The listing builds one solid part. Answer for the finished solid, in the listing's coordinates (mm). A direction names the side the tool comes from. Round coordinates to 2 decimals unless told otherwise and drop trailing zeros. Write each loop counter-clockwise with the first axis right and the second up, starting at its lowest first coordinate (ties: lowest second). Pieces come first, ordered by that corner, then holes. Notation, with made-up numbers: (3.5, 1.5) - (54.5, 1.5) arc R30 ccw to (54.5, 39.5) - close; hole circle Ø9 at (84, 18). An arc over 180 degrees is marked (long way). Return JSON: item names as keys, results as strings. Group by question number.
from build123d import *

# Parameters (mm, degrees)
SKETCH_1_W      = 148
SKETCH_1_H      = 22
SKETCH_1_W_2    = 10
SKETCH_1_H_2    = 3
EXTRUDE_1_DEPTH = 3


with BuildPart() as part:
    # 草图1 → 凸台-拉伸1 (new body)
    with BuildSketch(Plane.XY):
        Rectangle(SKETCH_1_W, SKETCH_1_H)
        with Locations((-52, 7.5)):
            Rectangle(SKETCH_1_W_2, SKETCH_1_H_2, mode=Mode.SUBTRACT)
        with Locations((-67, 7.5)):
            Rectangle(SKETCH_1_W_2, SKETCH_1_H_2, mode=Mode.SUBTRACT)
        with Locations((-37, 7.5)):
            Rectangle(SKETCH_1_W_2, SKETCH_1_H_2, mode=Mode.SUBTRACT)
        with Locations((-22, 7.5)):
            Rectangle(SKETCH_1_W_2, SKETCH_1_H_2, mode=Mode.SUBTRACT)
        with Locations((-7, 7.5)):
            Rectangle(SKETCH_1_W_2, SKETCH_1_H_2, mode=Mode.SUBTRACT)
        with Locations((8, 7.5)):
            Rectangle(SKETCH_1_W_2, SKETCH_1_H_2, mode=Mode.SUBTRACT)
        with Locations((23, 7.5)):
            Rectangle(SKETCH_1_W_2, SKETCH_1_H_2, mode=Mode.SUBTRACT)
        with Locations((38, 7.5)):
            Rectangle(SKETCH_1_W_2, SKETCH_1_H_2, mode=Mode.SUBTRACT)
        with Locations((53, 7.5)):
            Rectangle(SKETCH_1_W_2, SKETCH_1_H_2, mode=Mode.SUBTRACT)
        with Locations((68, 7.5)):
            Rectangle(SKETCH_1_W_2, SKETCH_1_H_2, mode=Mode.SUBTRACT)
        with Locations((68, -7.5)):
            Rectangle(SKETCH_1_W_2, SKETCH_1_H_2, mode=Mode.SUBTRACT)
        with Locations((53, -7.5)):
            Rectangle(SKETCH_1_W_2, SKETCH_1_H_2, mode=Mode.SUBTRACT)
        with Locations((38, -7.5)):
            Rectangle(SKETCH_1_W_2, SKETCH_1_H_2, mode=Mode.SUBTRACT)
        with Locations((23, -7.5)):
            Rectangle(SKETCH_1_W_2, SKETCH_1_H_2, mode=Mode.SUBTRACT)
        with Locations((8, -7.5)):
            Rectangle(SKETCH_1_W_2, SKETCH_1_H_2, mode=Mode.SUBTRACT)
        with Locations((-7, -7.5)):
            Rectangle(SKETCH_1_W_2, SKETCH_1_H_2, mode=Mode.SUBTRACT)
        with Locations((-22, -7.5)):
            Rectangle(SKETCH_1_W_2, SKETCH_1_H_2, mode=Mode.SUBTRACT)
        with Locations((-37, -7.5)):
            Rectangle(SKETCH_1_W_2, SKETCH_1_H_2, mode=Mode.SUBTRACT)
        with Locations((-52, -7.5)):
            Rectangle(SKETCH_1_W_2, SKETCH_1_H_2, mode=Mode.SUBTRACT)
        with Locations((-67, -7.5)):
            Rectangle(SKETCH_1_W_2, SKETCH_1_H_2, mode=Mode.SUBTRACT)
    extrude(amount=EXTRUDE_1_DEPTH)


solid = part.part
(1) Find section B-B (z = 2.5). State how many separate pieces and enclosed holes the cut face has, plus the area to 3 significant figures.
(2) For faces 1 (the flat face through (-1, 0, 3)), 2 (the flat face through (38, 6, 1)), determine the directions among +Z, -Z, +X, -X, +Y, -Y from which every point of the face is accessible in a straight line to the end or side of a thin tool.
(3) Consider line 1 (Y direction, x = 65, z = 2.3). Determine where the line is inside the solid, lowest interval first.
(4) Find section A-A (x = 50). Write down the section's boundary in (y, z).
Check sheet entries:
{
 "1": {"separate pieces": "1", "enclosed holes": "20", "area": "2,660 mm^2"},
 "2": {"face 1": "+Z, +X, -X, +Y, -Y", "face 2": "+Z, -Z"},
 "3": {"line 1": "y = -11 to -9, -6 to 6, 9 to 11"},
 "4": {"outline": "(-11, 0) - (-9, 0) - (-9, 3) - (-11, 3) - close; (-6, 0) - (6, 0) - (6, 3) - (-6, 3) - close; (9, 0) - (11, 0) - (11, 3) - (9, 3) - close"}
}
